For this review, take the finished solid that the model builds, in its own axes (mm). A direction names the side the tool comes from. Coordinates: 2 decimals unless noted, no trailing zeros. Loops run counter-clockwise (first coordinate to the right, second up) from the corner with the lowest first, then second, coordinate; pieces in that order, holes last.
Autodesk Inventor part; units mm, degrees
ref_plane "Work Plane1" through (1, 0, 0) normal (-1, 0, 0) x (0, 0, 1)
ref_plane "Work Plane2" through (1, 0, 0) normal (1, 0, 0) x (0, 0, -1)
ref_plane "YZ Plane" through (0, 0, 0) normal (1, 0, 0) x (0, 1, 0)
sketch "Sketch1" plane through (0, 0, 0) normal (0, 0, 1) x (1, 0, 0)
  line L0 (0, 0) -> (2, 0)
  line L1 (2, 0) -> (2, 2.75)
  line L2 (2, 2.75) -> (0, 2.75)
  line L3 (0, 2.75) -> (0, 0)
  line L4 (2, 0) -> (8, 0)
  line L5 (8, 0) -> (8, 1.95)
  line L6 (8, 1.95) -> (2, 1.95)
  line L7 (2, 1.95) -> (2, 0)
  dimension "d0" = 8
  dimension "d1" = 2
  dimension "d2" = 5.5
  dimension "d3" = 3.9
revolve "Revolution1" add sketch "Sketch1" angle 360 about axis through (0, 0, 0) along (1, 0, 0)
ref_plane "Work Plane1" through (1, 0, 0) normal (-1, 0, 0) x (0, 0, 1)
ref_plane "Work Plane2" through (1, 0, 0) normal (1, 0, 0) x (0, 0, -1)
sketch "Sketch2" plane through (0, 0, 0) normal (0, 0, 1) x (1, 0, 0)
  line L0 (0, 0.75) -> (1, 0.75)
  line L1 (1, 0.75) -> (1, -0.75)
  line L2 (1, -0.75) -> (0, -0.75)
  line L3 (0, -0.75) -> (0, 0.75)
  point P0 (0, 0)
  point P1 (0, 0)
  dimension "d7" = 1
  dimension "d8" = 1.5
extrude "Extrusion1" cut sketch "Sketch2" along normal through all both and the other way through all
hole "Hole1" at (8, 0, 0) direction (-1, 0, 0) diameter 2.013 depth 5 tip angle 118 counterbore diameter 3.5 counterbore depth 3
fillet "Fillet1" radius 0.12 4 edges at (0, 2.1937, -1.6583) (0, 2.1937, 1.6583) (0, -2.75, 0) (2, -2.75, 0)
properties part number "308-02" material "Steel"
Q1. Machinability: for faces 1 (the face through (1, 0, 0)), 2 (the face through (4.958, -1.437, -1.318)), 3 (the face through (0, -1, 0)), which of the approach directions +Z, -Z, +X, -X, +Y, -Y give a long, thin tool a straight path to every point of the face, cutting with its end or side? Answer none if there is none.
Q2. Consider section C-C (x = 4.5). State the section outline as (y, z) points, then the cut area to 3 significant figures.
Q3. The part is to be moulded in two halves that separate along Z. For faces 4 (the face through (0.99, 2.54, 1.05)), 5 (the face through (0.5, -0.75, 0)), 6 (the face through (5, 1, -1)), say which applies: +Z half, -Z half, draft (parallel to the pull), parting line (faces both ways), or undercut.
Q4. For pin 1 Ø0.5 at (y, z) = (0, 0) entering from -X; pin 2 Ø1 at (y, z) = (-1, -0.5) entering from +X; pin 3 Ø2 at (y, z) = (-1, -1) entering from +X; pin 4 Ø0.5 at (x, z) = (0.5, -1) entering from -Y, all flat-tipped, find the tip position at first contact; note any pin that passes through.
Q5. Wall thickness on probe 1 along Z at (x, y) = (6.5, 0); probe 2 along Z at (x, y) = (3.7, 0); probe 3 along X at (y, z) = (-1, -1.4): over which ranges is each line inside the solid? List them lowest first.
Q6. Consider section A-A (x = 7). State the section outline as (y, z) points, then the cut area to 3 significant figures.
Q7. Consider section B-B (x = 2.25). State the section outline as (y, z) points, then the cut area to 3 significant figures.
Model answer:
1. face 1: +Z, -Z, -X
1. face 2: +X
1. face 3: +Z, -Z, -X, +Y, -Y
2. outline: circle Ø3.9 at (0, 0); hole circle Ø2.01 at (0, 0)
2. area: 8.76 mm2
3. face 4: parting line
3. face 5: draft
3. face 6: undercut
4. pin 1: stops at x = 1
4. pin 2: stops at x = 5
4. pin 3: stops at x = 8
4. pin 4: stops at y = -2.65
5. probe 1: z = -1.95 to -1.75, 1.75 to 1.95
5. probe 2: z = -1.95 to -1.01, 1.01 to 1.95
5. probe 3: x = 0 to 5
6. outline: circle Ø3.9 at (0, 0); hole circle Ø3.5 at (0, 0)
6. area: 2.32 mm2
7. outline: circle Ø3.9 at (0, 0)
7. area: 11.9 mm2
